Part model, mm, in its own coordinate system. A direction names the side the tool comes from. Round coordinates to 2 decimals unless told otherwise and drop trailing zeros. Loops run counter-clockwise (first coordinate to the right, second up) from the corner with the lowest first, then second, coordinate; pieces in that order, holes last.
(1) Tool access for faces 1 (the face through (-13.09, 0.39, 0.92)), 2 (the face through (-18, 7, 2)), 3 (the face through (-18.398, 3.943, -0.106)): list every direction of +Z, -Z, +X, -X, +Y, -Y with a clear straight run to the whole face (end or side of a thin tool).
(2) Cut at A-A on x = -16. List the corners of the cut face in (y, z).
(3) Cut at C-C on y = 2.5. List the corners of the cut face in (x, z), then the cut area to 3 significant figures.
(4) Probe probe 1 along X at (y, z) = (7.5, 0); probe 2 along X at (y, z) = (2.75, 0); probe 3 along Z at (x, y) = (-16, 7.5). List the from-to ranges inside material, lowest first.
(5) Flat gauge pins, fed straight in: pin 1 (3 mm diameter, centred on x = -16, z = 0, fed in from +Y); pin 2 (1.5 mm diameter, centred on y = 1, z = 1, fed in from +X). Where does each tip first touch, or does it go through?
(6) Mould opens along X. For faces 4 (the face through (-13.09, 7.41, -0.92)), 5 (the face through (-18.9, 3.8, 2.3)) say: +X half, -X half, draft (parallel to the pull), parting line (faces both ways), or undercut.
(7) Cut at B-B on z = 0. List the corners of the cut face in (x, y).
from build123d import *

# Parameters (mm, degrees)
SKETCH1_R           = 3.7
BOSS_EXTRUDE3_DEPTH = 7.8
SKETCH2_R           = 2.4
CUT_EXTRUDE6_DEPTH  = 7.8
SKETCH3_R           = 3.05
CUT_EXTRUDE7_DEPTH  = 0.8
SKETCH4_R           = 3.05
CUT_EXTRUDE8_DEPTH  = 0.8


with BuildPart() as part:
    # Sketch1 → Boss-Extrude3 (new body)
    with BuildSketch(Plane(origin=(0, 0, 0), x_dir=(1, 0, 0), z_dir=(0, 1, 0))):
        with Locations((-16, 0)):
            Circle(SKETCH1_R)
    extrude(amount=BOSS_EXTRUDE3_DEPTH)

    # Sketch2 → Cut-Extrude6 (cut)
    with BuildSketch(Plane(origin=(0, 7.8, 0), x_dir=(1, 0, 0), z_dir=(0, 1, 0))):
        with Locations((-16, 0)):
            Circle(SKETCH2_R)
    extrude(amount=-CUT_EXTRUDE6_DEPTH, mode=Mode.SUBTRACT)

    # Sketch3 → Cut-Extrude7 (cut)
    with BuildSketch(Plane(origin=(0, 7.8, 0), x_dir=(1, 0, 0), z_dir=(0, 1, 0))):
        with Locations((-16, 0)):
            Circle(SKETCH3_R)
    extrude(amount=-CUT_EXTRUDE7_DEPTH, mode=Mode.SUBTRACT)

    # Sketch4 → Cut-Extrude8 (cut)
    with BuildSketch(Plane.XZ):
        with Locations((-16, 0)):
            Circle(SKETCH4_R)
    extrude(amount=-CUT_EXTRUDE8_DEPTH, mode=Mode.SUBTRACT)


solid = part.part
Final values:
1. face 1: -Y
1. face 2: +Y
1. face 3: +Y, -Y
2. outline: (0, -3.7) - (7.8, -3.7) - (7.8, -3.05) - (7, -3.05) - (7, -2.4) - (0.8, -2.4) - (0.8, -3.05) - (0, -3.05) - close; (0, 3.05) - (0.8, 3.05) - (0.8, 2.4) - (7, 2.4) - (7, 3.05) - (7.8, 3.05) - (7.8, 3.7) - (0, 3.7) - close
3. outline: circle Ø7.4 at (-16, 0); hole circle Ø4.8 at (-16, 0)
3. area: 24.9 mm2
4. probe 1: x = -19.7 to -19.05, -12.95 to -12.3
4. probe 2: x = -19.7 to -18.4, -13.6 to -12.3
4. probe 3: z = -3.7 to -3.05, 3.05 to 3.7
5. pin 1: passes through
5. pin 2: stops at x = -12.31
6. face 4: undercut
6. face 5: parting line
7. outline: (-19.7, 0) - (-19.05, 0) - (-19.05, 0.8) - (-18.4, 0.8) - (-18.4, 7) - (-19.05, 7) - (-19.05, 7.8) - (-19.7, 7.8) - close; (-13.6, 0.8) - (-12.95, 0.8) - (-12.95, 0) - (-12.3, 0) - (-12.3, 7.8) - (-12.95, 7.8) - (-12.95, 7) - (-13.6, 7) - close
